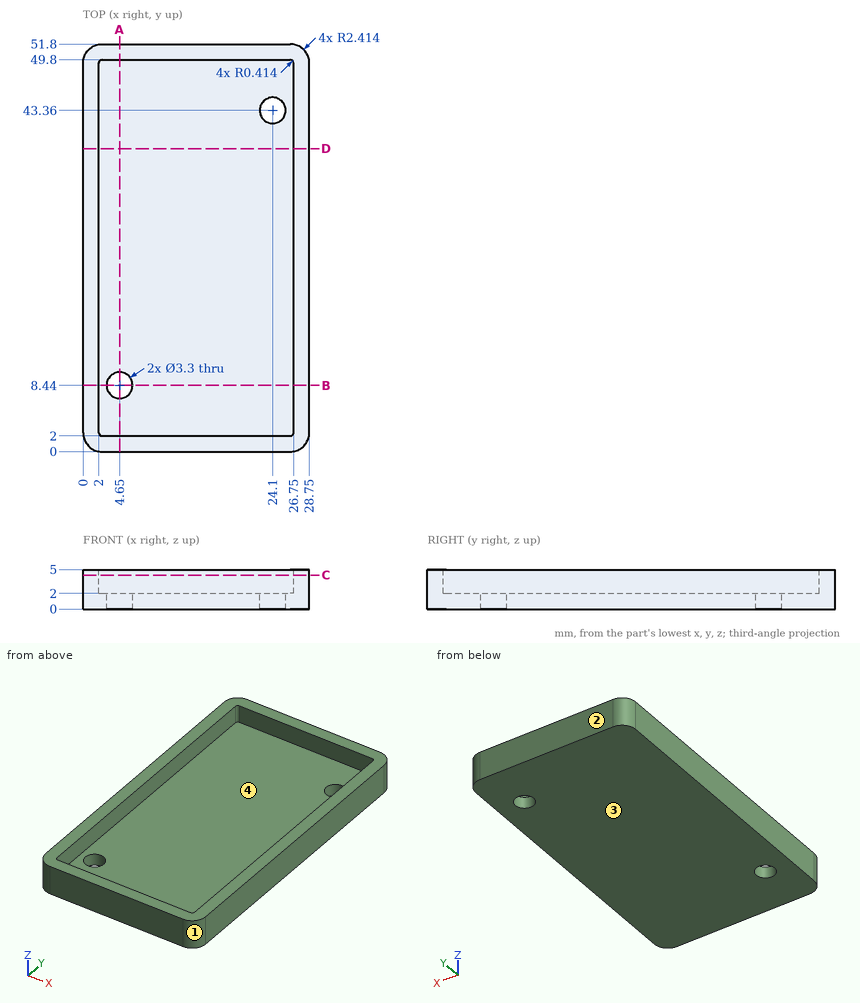
Could you check a few things on this drawing? It's one solid part, dimensions in mm from its lowest x, y, z. Round coordinates to 2 decimals unless told otherwise and drop trailing zeros. Write each loop counter-clockwise with the first axis right and the second up, starting at its lowest first coordinate (ties: lowest second). Pieces come first, ordered by that corner, then holes. Notation, with made-up numbers: (80.5, -28.5) -> (134.5, -28.5) arc R33 ccw to (134.5, 8.5) -> close; hole circle Ø9 at (-21.5, 18). An arc over 180 degrees is marked (long way). Use a Markdown table: item, result.
1. If we section it at B-B (y = 8.44): List the corners of the cut face in (x, z) for me.
Answer key:
| item | result |
|---|---|
| outline | (0, 0) -> (3, 0) -> (3, 2) -> (2, 2) -> (2, 5) -> (0, 5) -> close; (6.3, 0) -> (28.75, 0) -> (28.75, 5) -> (26.75, 5) -> (26.75, 2) -> (6.3, 2) -> close |
2. If we section it at A-A (x = 4.65): List the corners of the cut face in (y, z) for me.
Answer key:
| item | result |
|---|---|
| outline | (0, 0) -> (6.79, 0) -> (6.79, 2) -> (2, 2) -> (2, 5) -> (0, 5) -> close; (10.09, 0) -> (51.8, 0) -> (51.8, 5) -> (49.8, 5) -> (49.8, 2) -> (10.09, 2) -> close |
3. We'd pull the mould along Y, two halves only. Please class the marked faces 1, 2, 3 and 4: +Y half, -Y half, draft (parallel to the pull), parting line (faces both ways), or undercut.
Answer key:
| item | result |
|---|---|
| face 1 | -Y half |
| face 2 | +Y half |
| face 3 | draft |
| face 4 | undercut |
4. For pin 1 Ø7.5 at (x, y) = (19.5, 17.5) entering from +Z, with a flat end and sliding along its axis, tell me the tip position at first contact or that it passes through.
Answer key:
| item | result |
|---|---|
| pin 1 | stops at z = 2 |
5. If we section it at C-C (z = 4.3): List the corners of the cut face in (x, y) for me.
Answer key:
| item | result |
|---|---|
| outline | (0, 2.41) arc R2.41 ccw to (2.41, 0) -> (26.34, 0) arc R2.41 ccw to (28.75, 2.41) -> (28.75, 49.39) arc R2.41 ccw to (26.34, 51.8) -> (2.41, 51.8) arc R2.41 ccw to (0, 49.39) -> close; hole (2, 2.41) arc R0.41 ccw to (2.41, 2) -> (26.34, 2) arc R0.41 ccw to (26.75, 2.41) -> (26.75, 49.39) arc R0.41 ccw to (26.34, 49.8) -> (2.41, 49.8) arc R0.41 ccw to (2, 49.39) -> close |
6. Please list where these lines run through material, in increasing order: probe 1 along X at (y, z) = (8, 2.6); probe 2 along Y at (x, z) = (4.65, 0.85); probe 3 along Y at (x, z) = (6.75, 3.9).
Answer key:
| item | result |
|---|---|
| probe 1 | x = 0 to 2, 26.75 to 28.75 |
| probe 2 | y = 0 to 6.79, 10.09 to 51.8 |
| probe 3 | y = 0 to 2, 49.8 to 51.8 |
7. If we section it at D-D (y = 38.5): List the corners of the cut face in (x, z) for me, then the cut area to 3 significant figures.
Answer key:
| item | result |
|---|---|
| outline | (0, 0) -> (28.75, 0) -> (28.75, 5) -> (26.75, 5) -> (26.75, 2) -> (2, 2) -> (2, 5) -> (0, 5) -> close |
| area | 69.5 mm^2 |
